```python
from build123d import *

# Parameters (mm, degrees)
RETAINER_FEATURE_2_PROFILE_W = 14
RETAINER_FEATURE_2_PROFILE_H = 5
RETAINER_FEATURE_2_DEPTH     = 14
RETAINER_FEATURE_3_PROFILE_R = 3
RETAINER_FEATURE_3_DEPTH     = 3
RETAINER_FEATURE_4_PROFILE_R = 3
RETAINER_FEATURE_4_DEPTH     = 3
RETAINER_FEATURE_6_PROFILE_R = 1.1
RETAINER_FEATURE_6_DEPTH     = 4.25
RETAINER_FEATURE_7_PROFILE_R = 2.1
RETAINER_FEATURE_7_DEPTH     = 1.45
RETAINER_FEATURE_8_PROFILE_R = 1.1
RETAINER_FEATURE_8_DEPTH     = 4.25
RETAINER_FEATURE_9_PROFILE_R = 2.1
RETAINER_FEATURE_9_DEPTH     = 1.45
RETAINER_FEATURE_12_DEPTH    = 10


with BuildPart() as part:
    # Retainer Feature 1 profile → Retainer Feature 1 (revolve)
    with BuildSketch(Plane(origin=(0, -73, 0), x_dir=(-1, 0, 0), z_dir=(0, -1, 0))):
        with BuildLine():
            Line((26.291651246, -6), (26.291651246, 6))
            ThreePointArc((26.291651246, 6), (20.291651246, 0), (26.291651246, -6))
        make_face()
    revolve(axis=Axis((-26.291651246, -73, -10), (0, 0, 1)))

    # Retainer Feature 2 profile → Retainer Feature 2 (cut)
    with BuildSketch(Plane.XY.offset(-7)):
        with Locations((-26.291651246, -68.5)):
            Rectangle(RETAINER_FEATURE_2_PROFILE_W, RETAINER_FEATURE_2_PROFILE_H)
    extrude(amount=RETAINER_FEATURE_2_DEPTH, mode=Mode.SUBTRACT)

    # Retainer Feature 3 profile → Retainer Feature 3 (add)
    with BuildSketch(Plane(origin=(0, -71, 0), x_dir=(-1, 0, 0), z_dir=(0, -1, 0))):
        with Locations((26.291651246, 8.5)):
            Circle(RETAINER_FEATURE_3_PROFILE_R)
    extrude(amount=RETAINER_FEATURE_3_DEPTH)

    # Retainer Feature 4 profile → Retainer Feature 4 (add)
    with BuildSketch(Plane(origin=(0, -71, 0), x_dir=(-1, 0, 0), z_dir=(0, -1, 0))):
        with Locations((26.291651246, -8.5)):
            Circle(RETAINER_FEATURE_4_PROFILE_R)
    extrude(amount=RETAINER_FEATURE_4_DEPTH)

    # Retainer Feature 5 profile → Retainer Feature 5 (revolve, cut)
    with BuildSketch(Plane(origin=(0, -73, 0), x_dir=(-1, 0, 0), z_dir=(0, -1, 0))):
        with BuildLine():
            Line((26.291651246, -3.15), (26.291651246, 3.15))
            ThreePointArc((26.291651246, 3.15), (23.141651246, 0), (26.291651246, -3.15))
        make_face()
    revolve(axis=Axis((-26.291651246, -73, -10), (0, 0, 1)), mode=Mode.SUBTRACT)

    # Retainer Feature 6 profile → Retainer Feature 6 (cut)
    with BuildSketch(Plane(origin=(0, -70, 0), x_dir=(-1, 0, 0), z_dir=(0, -1, 0))):
        with Locations(Location((26.291651246, 8.5, 0), (0, 0, 270))):
            Circle(RETAINER_FEATURE_6_PROFILE_R)
    extrude(amount=RETAINER_FEATURE_6_DEPTH, mode=Mode.SUBTRACT)

    # Retainer Feature 7 profile → Retainer Feature 7 (cut)
    with BuildSketch(Plane(origin=(0, -72.8, 0), x_dir=(-1, 0, 0), z_dir=(0, -1, 0))):
        with Locations(Location((26.291651246, 8.5, 0), (0, 0, 90))):
            Circle(RETAINER_FEATURE_7_PROFILE_R)
    extrude(amount=RETAINER_FEATURE_7_DEPTH, mode=Mode.SUBTRACT)

    # Retainer Feature 8 profile → Retainer Feature 8 (cut)
    with BuildSketch(Plane(origin=(0, -70, 0), x_dir=(-1, 0, 0), z_dir=(0, -1, 0))):
        with Locations(Location((26.291651246, -8.5, 0), (0, 0, 270))):
            Circle(RETAINER_FEATURE_8_PROFILE_R)
    extrude(amount=RETAINER_FEATURE_8_DEPTH, mode=Mode.SUBTRACT)

    # Retainer Feature 9 profile → Retainer Feature 9 (cut)
    with BuildSketch(Plane(origin=(0, -72.8, 0), x_dir=(-1, 0, 0), z_dir=(0, -1, 0))):
        with Locations(Location((26.291651246, -8.5, 0), (0, 0, 90))):
            Circle(RETAINER_FEATURE_9_PROFILE_R)
    extrude(amount=RETAINER_FEATURE_9_DEPTH, mode=Mode.SUBTRACT)

    # Middle Right Fixed Compression Ball Reta → Retainer Feature 12 (cut)
    with BuildSketch(Plane(origin=(-46.801806266, -32.220261504, -18.815460044), x_dir=(-0.25892602820646665, -0.17825517869277457, 0.9493062747008634), z_dir=(-0.7819246728070284, -0.5383086561091627, -0.3143526631246647))):
        Polygon((20.297287002, -41.528985171), (16.35135873, -46.567799523), (19.343154751, -48.910694434), (23.289083023, -43.871880083), align=None)
    extrude(amount=RETAINER_FEATURE_12_DEPTH, mode=Mode.SUBTRACT)


solid = part.part
```
Part model, mm, in its own coordinate system. A direction names the side the tool comes from. Coordinates: 2 decimals unless noted, no trailing zeros. Loops run counter-clockwise (first coordinate to the right, second up) from the corner with the lowest first, then second, coordinate; pieces in that order, holes last. Notation, with made-up numbers: (30.25, -13.75) - (71.25, -13.75) arc R13 ccw to (71.25, -4.75) - close; hole circle Ø6 at (30.5, 60). An arc over 180 degrees is marked (long way). Write item = value, one per line. Start each with the question number.
Item 1: Cut at A-A, the plane z = -8.5. Give the cut face in (x, y), and give its area (3 significant figures).
Item 2: Flat gauge pins, fed straight in: pin 1 Ø1.3 at (x, z) = (-27.5, -8) entering from -Y; pin 2 Ø6 at (x, z) = (-30.5, 7) entering from +Y; pin 3 Ø1.5 at (y, z) = (-68.5, 6) entering from +X; pin 4 Ø5 at (x, z) = (-22.5, 0) entering from -Y. Where does each tip first touch, or does it go through?
Item 3: Cut at D-D, the plane x = -22.75. Give the cut face in (y, z).
Item 4: Wall check: L1, parallel to X at y = -73.45, z = 8.5; L2, parallel to X at y = -71.5, z = -8.5; L3, parallel to Z at x = -25.25, y = -73.5. Give the ranges that are in metal, low to high. Write a range as from..to.
Item 5: Mould opens along Y. For faces 4 (the flat face through (-26, -74, 11)), 5 (the cylindrical face through (-27.569, -73.392, 10.166)), 6 (the flat face through (-28.68, -76.11, 0.31)) say: released by +Y, released by -Y, zero draft, split by the parting line, or undercut.
Item 6: 3-axis set-ups, long thin cutter, end or side, ignore diameter. For faces 1 (the cylindrical face through (-27.382, -71.887, -8.643)), 2 (the flat face through (-30.18, -72.64, 1.11)), 3 (the cylindrical face through (-28.34, -73.39, -8.04)): which of +Z, -Z, +X, -X, +Y, -Y reach the whole face in a straight line?
Item 7: Cut at C-C, the plane z = -4.5. Give the cut face in (x, y), and give its area (3 significant figures).
Item 8: Cut at B-B, the plane y = -72.25. Give the cut face in (x, z), and give its area (3 significant figures).
The answers:
q1.outline = (-29.29, -74) - (-28.39, -74) - (-28.39, -72.8) - (-27.39, -72.8) - (-27.39, -71) - (-29.29, -71) - close; (-25.19, -72.8) - (-24.19, -72.8) - (-24.19, -74) - (-23.29, -74) - (-23.29, -71) - (-25.19, -71) - close
q1.area = 9.00 mm2
q2.pin_1 = -72.8
q2.pin_2 = -71
q2.pin_3 = through
q2.pin_4 = -78.86
q3.outline = (-71, -4.41) - (-71, 4.41) arc R4.84 ccw (long way) to start
q4.L1 = -29.29..-28.39, -24.19..-23.29
q4.L2 = -29.29..-27.39, -25.19..-23.29
q4.L3 = -11.31..-10.32, -6.68..-3.18, 2.93..6.68, 10.32..11.31
q5.face_4 = released by -Y
q5.face_5 = zero draft
q5.face_6 = undercut
q6.face_1 = +Y, -Y
q6.face_2 = none
q6.face_3 = -Y
q7.outline = (-29.72, -71) arc R3.97 ccw to (-29.03, -75.87) - (-27.63, -75.56) - (-28.36, -76.38) arc R3.97 ccw to (-22.86, -71) - close
q7.area = 39.4 mm2
q8.outline = (-27.61, -5.81) arc R3 ccw (long way) to (-24.97, -5.81) arc R5.95 ccw to (-24.97, 5.81) arc R3 ccw (long way) to (-27.61, 5.81) arc R5.95 ccw to start; hole (-31.71, -0.83) - (-29.03, -1.36) arc R3.06 ccw (long way) to (-27.86, 2.62) - (-28.01, 3) - close; hole circle Ø2.2 at (-26.29, -8.5); hole circle Ø2.2 at (-26.29, 8.5)
q8.area = 125 mm2
